Design review of the part built by this model. Coordinates are the model's own, in mm. Coordinates: 2 decimals unless noted, no trailing zeros. Write each loop counter-clockwise with the first axis right and the second up, starting at its lowest first coordinate (ties: lowest second). Pieces come first, ordered by that corner, then holes. Notation, with made-up numbers: (3, 81.25) -> (8, 81.25) arc R18 cw to (8, 90.25) -> close; hole circle Ø8 at (5, 67.25). An arc over 180 degrees is marked (long way). One line per question, with ' | ' between items. Start each with the question number.
Q1. Add section D-D on z = 1.4. Give the number of separate pieces and of enclosed holes in the cut face, and give its area (3 significant figures).
Q2. Add section A-A on x = -13. State the section outline as (y, z) points, and give its area (3 significant figures).
Q3. For P1, Ø2.5, axis at y = 15, z = 2, coming from the -X side; P2, Ø2.5, axis at x = -35.5, y = 10, coming from the +Z side, all flat-tipped, find the tip position at first contact; note any pin that passes through.
Q4. Add section B-B on x = -53.1. State the section outline as (y, z) points (3 decimals), and give its area (3 significant figures).
Q5. Wall thickness on probe 1 along X at (y, z) = (12, 1.8); probe 2 along Y at (x, z) = (53.1, 3.25) (3 decimals); probe 3 along X at (y, z) = (-2, 0.7) (3 decimals): over which ranges is each line inside the solid? List them lowest first.
Q6. Add section C-C on y = 0. State the section outline as (x, z) points (3 decimals).
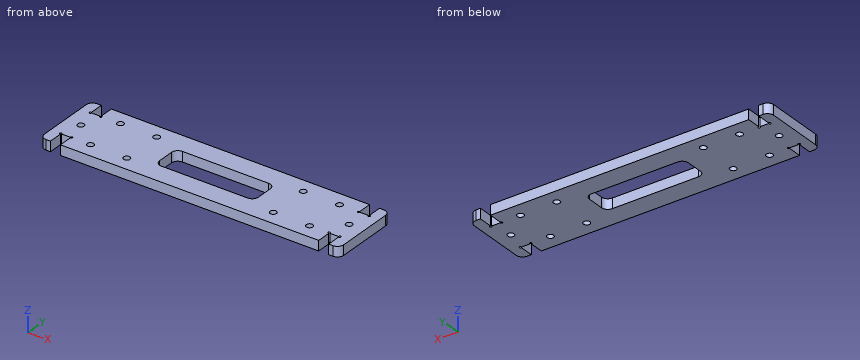
from build123d import *

# Parameters (mm, degrees)
F0_W      = 145
F0_H      = 34
F1_DEPTH  = 4.826
F2_R      = 1.575
F3_DEPTH  = 4.826
F4_R      = 3
F5_W      = 4.826
F5_H      = 7
F5_R      = 1.55
F6_DEPTH  = 4.827
F7_R      = 0.5
F8_DEPTH  = 4.827
F9_W      = 47.85
F9_H      = 14
F10_DEPTH = 4.827
F11_R     = 3


with BuildPart() as f1:
    # F0 (on Top) → F1 (new body)
    with BuildSketch(Plane.XY):
        Rectangle(F0_W, F0_H)
    extrude(amount=F1_DEPTH)

    # F2 (on face) → F3 (cut, through all)
    with BuildSketch(Plane.XY.offset(4.826)):
        with Locations((-53.1, -10)):
            Circle(F2_R)
        with Locations((-35.5, -10)):
            Circle(F2_R)
        with Locations((53.1, -10)):
            Circle(F2_R)
        with Locations((35.5, -10)):
            Circle(F2_R)
        with Locations((-35.5, 10)):
            Circle(F2_R)
        with Locations((-53.1, 10)):
            Circle(F2_R)
        with Locations((35.5, 10)):
            Circle(F2_R)
        with Locations((53.1, 10)):
            Circle(F2_R)
    extrude(amount=-F3_DEPTH, mode=Mode.SUBTRACT)

    # F4
    f4_edges = [f1.edges().sort_by_distance(p)[0] for p in [
        (-72.5, -17, 2.413),
        (-72.5, 17, 2.413),
        (72.5, -17, 2.413),
        (72.5, 17, 2.413),
    ]]
    fillet(f4_edges, radius=F4_R)

    # F5 (on face) → F6 (cut, through all)
    with BuildSketch(Plane.XY.offset(4.826)):
        with Locations((-65, 13.5)):
            Rectangle(F5_W, F5_H)
        with Locations((-65, -13.5)):
            Rectangle(F5_W, F5_H)
        with Locations((-65, 0)):
            Circle(F5_R)
        with Locations((65, -13.5)):
            Rectangle(F5_W, F5_H)
        with Locations((65, 13.5)):
            Rectangle(F5_W, F5_H)
        with Locations((65, 0)):
            Circle(F5_R)
    extrude(amount=-F6_DEPTH, mode=Mode.SUBTRACT)

    # F7 (on face) → F8 (cut, through all)
    with BuildSketch(Plane.XY.offset(4.826)):
        with Locations((-67.589777, 9.823223)):
            Circle(F7_R)
        with Locations((-62.410223, 9.823223)):
            Circle(F7_R)
        with Locations((-67.589777, -9.823223)):
            Circle(F7_R)
        with Locations((-62.410223, -9.823223)):
            Circle(F7_R)
        with Locations((67.589777, 9.823223)):
            Circle(F7_R)
        with Locations((62.410223, 9.823223)):
            Circle(F7_R)
        with Locations((62.410223, -9.823223)):
            Circle(F7_R)
        with Locations((67.589777, -9.823223)):
            Circle(F7_R)
    extrude(amount=-F8_DEPTH, mode=Mode.SUBTRACT)

    # F9 (on face) → F10 (cut, through all)
    with BuildSketch(Plane.XY.offset(4.826)):
        Rectangle(F9_W, F9_H)
    extrude(amount=-F10_DEPTH, mode=Mode.SUBTRACT)

    # F11
    f11_edges = [f1.edges().sort_by_distance(p)[0] for p in [
        (-23.925, 7, 2.413),
        (-23.925, -7, 2.413),
        (23.925, 7, 2.413),
        (23.925, -7, 2.413),
    ]]
    fillet(f11_edges, radius=F11_R)


solid = f1.part
Output values:
1) separate pieces: 1 | enclosed holes: 11 | area: 4,040 mm2
2) outline: (-17, 0) -> (-7, 0) -> (-7, 4.83) -> (-17, 4.83) -> close; (7, 0) -> (17, 0) -> (17, 4.83) -> (7, 4.83) -> close | area: 96.5 mm2
3) P1: stops at x = -72.5 | P2: passes through
4) outline: (-17, 0) -> (-11.575, 0) -> (-11.575, 4.826) -> (-17, 4.826) -> close; (-8.425, 0) -> (8.425, 0) -> (8.425, 4.826) -> (-8.425, 4.826) -> close; (11.575, 0) -> (17, 0) -> (17, 4.826) -> (11.575, 4.826) -> close | area: 134 mm2
5) probe 1: x = -72.5 to -67.41, -62.59 to 62.59, 67.41 to 72.5 | probe 2: y = -17 to -11.575, -8.425 to 8.425, 11.575 to 17 | probe 3: x = -72.5 to -23.925, 23.925 to 72.5
6) outline: (-72.5, 0) -> (-66.55, 0) -> (-66.55, 4.826) -> (-72.5, 4.826) -> close; (-63.45, 0) -> (-23.925, 0) -> (-23.925, 4.826) -> (-63.45, 4.826) -> close; (23.925, 0) -> (63.45, 0) -> (63.45, 4.826) -> (23.925, 4.826) -> close; (66.55, 0) -> (72.5, 0) -> (72.5, 4.826) -> (66.55, 4.826) -> close
